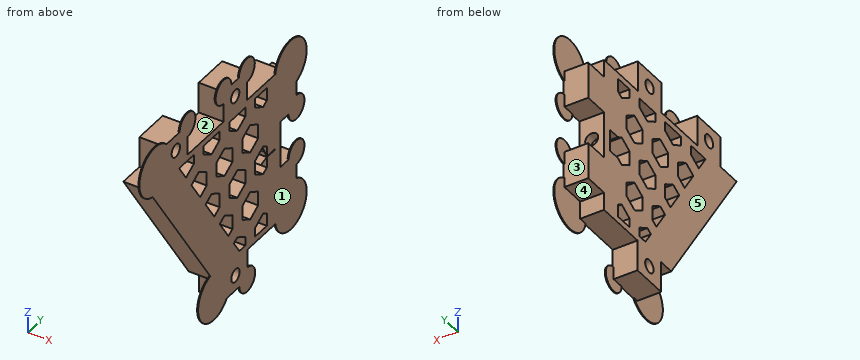
from build123d import *

# Parameters (mm, degrees)
HONEYCOMB_W      = 109
HONEYCOMB_H      = 99.592922
EXTRUDE002_DEPTH = 8
PAD002_DEPTH     = 8
PAD001_DEPTH     = 5.1
PAD_DEPTH        = 8
SKETCH001_W      = 8.1
SKETCH001_H      = 10
SKETCH001_W_2    = 18.2
SKETCH001_W_3    = 5.1
SKETCH001_W_4    = 8
SKETCH001_H_2    = 15.2
POCKET_DEPTH     = 8.001
SKETCH002_R      = 2.1
POCKET001_DEPTH  = 8.001
SKETCH004_R      = 2.1
POCKET002_DEPTH  = 7
SKETCH006_R      = 8
SKETCH006_R_2    = 4
PAD003_DEPTH     = 0.3


with BuildPart() as extrude002:
    # Honeycomb → Extrude002 (new body)
    with BuildSketch(Plane(origin=(0, 0, -0.165735), x_dir=(0, -1, 0), z_dir=(1, 0, 0))):
        with Locations((0, -0.165735)):
            Rectangle(HONEYCOMB_W, HONEYCOMB_H)
        Polygon((41.5, -37.26049), (45.5, -34.951089), (49.5, -37.26049), (49.5, -41.879292), (45.5, -44.188693), (41.5, -41.879292), align=None, mode=Mode.SUBTRACT)
        Polygon((28.5, -37.26049), (32.5, -34.951089), (36.5, -37.26049), (36.5, -41.879292), (32.5, -44.188693), (28.5, -41.879292), align=None, mode=Mode.SUBTRACT)
        Polygon((15.5, -37.26049), (19.5, -34.951089), (23.5, -37.26049), (23.5, -41.879292), (19.5, -44.188693), (15.5, -41.879292), align=None, mode=Mode.SUBTRACT)
        Polygon((2.5, -37.26049), (6.5, -34.951089), (10.5, -37.26049), (10.5, -41.879292), (6.5, -44.188693), (2.5, -41.879292), align=None, mode=Mode.SUBTRACT)
        Polygon((-10.5, -37.26049), (-6.5, -34.951089), (-2.5, -37.26049), (-2.5, -41.879292), (-6.5, -44.188693), (-10.5, -41.879292), align=None, mode=Mode.SUBTRACT)
        Polygon((-23.5, -37.26049), (-19.5, -34.951089), (-15.5, -37.26049), (-15.5, -41.879292), (-19.5, -44.188693), (-23.5, -41.879292), align=None, mode=Mode.SUBTRACT)
        Polygon((-36.5, -37.26049), (-32.5, -34.951089), (-28.5, -37.26049), (-28.5, -41.879292), (-32.5, -44.188693), (-36.5, -41.879292), align=None, mode=Mode.SUBTRACT)
        Polygon((-49.5, -37.26049), (-45.5, -34.951089), (-41.5, -37.26049), (-41.5, -41.879292), (-45.5, -44.188693), (-49.5, -41.879292), align=None, mode=Mode.SUBTRACT)
        Polygon((35, -26.00216), (39, -23.692759), (43, -26.00216), (43, -30.620962), (39, -32.930363), (35, -30.620962), align=None, mode=Mode.SUBTRACT)
        Polygon((22, -26.00216), (26, -23.692759), (30, -26.00216), (30, -30.620962), (26, -32.930363), (22, -30.620962), align=None, mode=Mode.SUBTRACT)
        Polygon((9, -26.00216), (13, -23.692759), (17, -26.00216), (17, -30.620962), (13, -32.930363), (9, -30.620962), align=None, mode=Mode.SUBTRACT)
        Polygon((-4, -26.00216), (0, -23.692759), (4, -26.00216), (4, -30.620962), (0, -32.930363), (-4, -30.620962), align=None, mode=Mode.SUBTRACT)
        Polygon((-17, -26.00216), (-13, -23.692759), (-9, -26.00216), (-9, -30.620962), (-13, -32.930363), (-17, -30.620962), align=None, mode=Mode.SUBTRACT)
        Polygon((-30, -26.00216), (-26, -23.692759), (-22, -26.00216), (-22, -30.620962), (-26, -32.930363), (-30, -30.620962), align=None, mode=Mode.SUBTRACT)
        Polygon((-43, -26.00216), (-39, -23.692759), (-35, -26.00216), (-35, -30.620962), (-39, -32.930363), (-43, -30.620962), align=None, mode=Mode.SUBTRACT)
        Polygon((41.5, -14.743829), (45.5, -12.434428), (49.5, -14.743829), (49.5, -19.362632), (45.5, -21.672033), (41.5, -19.362632), align=None, mode=Mode.SUBTRACT)
        Polygon((28.5, -14.743829), (32.5, -12.434428), (36.5, -14.743829), (36.5, -19.362632), (32.5, -21.672033), (28.5, -19.362632), align=None, mode=Mode.SUBTRACT)
        Polygon((15.5, -14.743829), (19.5, -12.434428), (23.5, -14.743829), (23.5, -19.362632), (19.5, -21.672033), (15.5, -19.362632), align=None, mode=Mode.SUBTRACT)
        Polygon((2.5, -14.743829), (6.5, -12.434428), (10.5, -14.743829), (10.5, -19.362632), (6.5, -21.672033), (2.5, -19.362632), align=None, mode=Mode.SUBTRACT)
        Polygon((-10.5, -14.743829), (-6.5, -12.434428), (-2.5, -14.743829), (-2.5, -19.362632), (-6.5, -21.672033), (-10.5, -19.362632), align=None, mode=Mode.SUBTRACT)
        Polygon((-23.5, -14.743829), (-19.5, -12.434428), (-15.5, -14.743829), (-15.5, -19.362632), (-19.5, -21.672033), (-23.5, -19.362632), align=None, mode=Mode.SUBTRACT)
        Polygon((-36.5, -14.743829), (-32.5, -12.434428), (-28.5, -14.743829), (-28.5, -19.362632), (-32.5, -21.672033), (-36.5, -19.362632), align=None, mode=Mode.SUBTRACT)
        Polygon((-49.5, -14.743829), (-45.5, -12.434428), (-41.5, -14.743829), (-41.5, -19.362632), (-45.5, -21.672033), (-49.5, -19.362632), align=None, mode=Mode.SUBTRACT)
        Polygon((35, -3.485499), (39, -1.176098), (43, -3.485499), (43, -8.104301), (39, -10.413702), (35, -8.104301), align=None, mode=Mode.SUBTRACT)
        Polygon((22, -3.485499), (26, -1.176098), (30, -3.485499), (30, -8.104301), (26, -10.413702), (22, -8.104301), align=None, mode=Mode.SUBTRACT)
        Polygon((9, -3.485499), (13, -1.176098), (17, -3.485499), (17, -8.104301), (13, -10.413702), (9, -8.104301), align=None, mode=Mode.SUBTRACT)
        Polygon((-4, -3.485499), (0, -1.176098), (4, -3.485499), (4, -8.104301), (0, -10.413702), (-4, -8.104301), align=None, mode=Mode.SUBTRACT)
        Polygon((-17, -3.485499), (-13, -1.176098), (-9, -3.485499), (-9, -8.104301), (-13, -10.413702), (-17, -8.104301), align=None, mode=Mode.SUBTRACT)
        Polygon((-30, -3.485499), (-26, -1.176098), (-22, -3.485499), (-22, -8.104301), (-26, -10.413702), (-30, -8.104301), align=None, mode=Mode.SUBTRACT)
        Polygon((-43, -3.485499), (-39, -1.176098), (-35, -3.485499), (-35, -8.104301), (-39, -10.413702), (-43, -8.104301), align=None, mode=Mode.SUBTRACT)
        Polygon((41.5, 7.772831), (45.5, 10.082232), (49.5, 7.772831), (49.5, 3.154029), (45.5, 0.844628), (41.5, 3.154029), align=None, mode=Mode.SUBTRACT)
        Polygon((28.5, 7.772831), (32.5, 10.082232), (36.5, 7.772831), (36.5, 3.154029), (32.5, 0.844628), (28.5, 3.154029), align=None, mode=Mode.SUBTRACT)
        Polygon((15.5, 7.772831), (19.5, 10.082232), (23.5, 7.772831), (23.5, 3.154029), (19.5, 0.844628), (15.5, 3.154029), align=None, mode=Mode.SUBTRACT)
        Polygon((2.5, 7.772831), (6.5, 10.082232), (10.5, 7.772831), (10.5, 3.154029), (6.5, 0.844628), (2.5, 3.154029), align=None, mode=Mode.SUBTRACT)
        Polygon((-10.5, 7.772831), (-6.5, 10.082232), (-2.5, 7.772831), (-2.5, 3.154029), (-6.5, 0.844628), (-10.5, 3.154029), align=None, mode=Mode.SUBTRACT)
        Polygon((-23.5, 7.772831), (-19.5, 10.082232), (-15.5, 7.772831), (-15.5, 3.154029), (-19.5, 0.844628), (-23.5, 3.154029), align=None, mode=Mode.SUBTRACT)
        Polygon((-36.5, 7.772831), (-32.5, 10.082232), (-28.5, 7.772831), (-28.5, 3.154029), (-32.5, 0.844628), (-36.5, 3.154029), align=None, mode=Mode.SUBTRACT)
        Polygon((-49.5, 7.772831), (-45.5, 10.082232), (-41.5, 7.772831), (-41.5, 3.154029), (-45.5, 0.844628), (-49.5, 3.154029), align=None, mode=Mode.SUBTRACT)
        Polygon((35, 19.031161), (39, 21.340562), (43, 19.031161), (43, 14.412359), (39, 12.102958), (35, 14.412359), align=None, mode=Mode.SUBTRACT)
        Polygon((22, 19.031161), (26, 21.340562), (30, 19.031161), (30, 14.412359), (26, 12.102958), (22, 14.412359), align=None, mode=Mode.SUBTRACT)
        Polygon((9, 19.031161), (13, 21.340562), (17, 19.031161), (17, 14.412359), (13, 12.102958), (9, 14.412359), align=None, mode=Mode.SUBTRACT)
        Polygon((-4, 19.031161), (0, 21.340562), (4, 19.031161), (4, 14.412359), (0, 12.102958), (-4, 14.412359), align=None, mode=Mode.SUBTRACT)
        Polygon((-17, 19.031161), (-13, 21.340562), (-9, 19.031161), (-9, 14.412359), (-13, 12.102958), (-17, 14.412359), align=None, mode=Mode.SUBTRACT)
        Polygon((-30, 19.031161), (-26, 21.340562), (-22, 19.031161), (-22, 14.412359), (-26, 12.102958), (-30, 14.412359), align=None, mode=Mode.SUBTRACT)
        Polygon((-43, 19.031161), (-39, 21.340562), (-35, 19.031161), (-35, 14.412359), (-39, 12.102958), (-43, 14.412359), align=None, mode=Mode.SUBTRACT)
        Polygon((41.5, 30.289492), (45.5, 32.598893), (49.5, 30.289492), (49.5, 25.670689), (45.5, 23.361288), (41.5, 25.670689), align=None, mode=Mode.SUBTRACT)
        Polygon((28.5, 30.289492), (32.5, 32.598893), (36.5, 30.289492), (36.5, 25.670689), (32.5, 23.361288), (28.5, 25.670689), align=None, mode=Mode.SUBTRACT)
        Polygon((15.5, 30.289492), (19.5, 32.598893), (23.5, 30.289492), (23.5, 25.670689), (19.5, 23.361288), (15.5, 25.670689), align=None, mode=Mode.SUBTRACT)
        Polygon((2.5, 30.289492), (6.5, 32.598893), (10.5, 30.289492), (10.5, 25.670689), (6.5, 23.361288), (2.5, 25.670689), align=None, mode=Mode.SUBTRACT)
        Polygon((-10.5, 30.289492), (-6.5, 32.598893), (-2.5, 30.289492), (-2.5, 25.670689), (-6.5, 23.361288), (-10.5, 25.670689), align=None, mode=Mode.SUBTRACT)
        Polygon((-23.5, 30.289492), (-19.5, 32.598893), (-15.5, 30.289492), (-15.5, 25.670689), (-19.5, 23.361288), (-23.5, 25.670689), align=None, mode=Mode.SUBTRACT)
        Polygon((-36.5, 30.289492), (-32.5, 32.598893), (-28.5, 30.289492), (-28.5, 25.670689), (-32.5, 23.361288), (-36.5, 25.670689), align=None, mode=Mode.SUBTRACT)
        Polygon((-49.5, 30.289492), (-45.5, 32.598893), (-41.5, 30.289492), (-41.5, 25.670689), (-45.5, 23.361288), (-49.5, 25.670689), align=None, mode=Mode.SUBTRACT)
        Polygon((35, 41.547822), (39, 43.857223), (43, 41.547822), (43, 36.92902), (39, 34.619619), (35, 36.92902), align=None, mode=Mode.SUBTRACT)
        Polygon((22, 41.547822), (26, 43.857223), (30, 41.547822), (30, 36.92902), (26, 34.619619), (22, 36.92902), align=None, mode=Mode.SUBTRACT)
        Polygon((9, 41.547822), (13, 43.857223), (17, 41.547822), (17, 36.92902), (13, 34.619619), (9, 36.92902), align=None, mode=Mode.SUBTRACT)
        Polygon((-4, 41.547822), (0, 43.857223), (4, 41.547822), (4, 36.92902), (0, 34.619619), (-4, 36.92902), align=None, mode=Mode.SUBTRACT)
        Polygon((-17, 41.547822), (-13, 43.857223), (-9, 41.547822), (-9, 36.92902), (-13, 34.619619), (-17, 36.92902), align=None, mode=Mode.SUBTRACT)
        Polygon((-30, 41.547822), (-26, 43.857223), (-22, 41.547822), (-22, 36.92902), (-26, 34.619619), (-30, 36.92902), align=None, mode=Mode.SUBTRACT)
        Polygon((-43, 41.547822), (-39, 43.857223), (-35, 41.547822), (-35, 36.92902), (-39, 34.619619), (-43, 36.92902), align=None, mode=Mode.SUBTRACT)
    extrude(amount=EXTRUDE002_DEPTH)


with BuildPart() as extrude002_1:
    # Extrude002 placement: moved
    add(extrude002.part.moved(Location((0, 1.1, 5.6))))


with BuildPart() as common:
    # Sketch005 → Pad002 (new body)
    with BuildSketch(Plane.YZ):
        Polygon((22.5, 23.15), (22.5, -23.15), (8.5944, -23.15), (-21.8273, 23.15), align=None)
    extrude(amount=PAD002_DEPTH)

    # Common: intersect Extrude002
    add(extrude002_1.part, mode=Mode.INTERSECT)


with BuildPart() as pad001:
    # Sketch003 → Pad001 (new body)
    with BuildSketch(Plane.XZ.offset(-26.5)):
        Polygon((1.96484, -3.525), (6.03516, -3.525), (8.070319, 0), (6.03516, 3.525), (0, 3.525), (0, -3.525), align=None)
    extrude(amount=PAD001_DEPTH)


with BuildPart() as obj1:
    # Sketch → Pad (new body)
    with BuildSketch(Plane.YZ):
        Polygon((-37.5, 35.15), (37.5, 35.15), (37.5, -35.15), (-4.45, -35.15), (-4.45, -25.15), (-37.5, 25.15), align=None)
        Polygon((-21.827321, 23.15), (22.5, 23.15), (22.5, -23.15), (8.594449, -23.15), align=None, mode=Mode.SUBTRACT)
    extrude(amount=PAD_DEPTH)

    # Sketch001 → Pocket (cut, through all)
    with BuildSketch(Plane.YZ.offset(8)):
        with Locations((-33.45, 30.15)):
            Rectangle(SKETCH001_W, SKETCH001_H)
        with Locations((-8.5, 30.15)):
            Rectangle(SKETCH001_W_2, SKETCH001_H)
        Polygon((37.5, 35.15), (12.4, 35.15), (12.4, 25.15), (29.5, 25.15), (29.5, 19.45), (37.5, 19.45), align=None)
        with Locations((-1.9, -30.15)):
            Rectangle(SKETCH001_W_3, SKETCH001_H)
        Polygon((12.6, -35.15), (37.5, -35.15), (37.5, -25.15), (37.5, -19.4), (29.5, -19.4), (29.5, -25.15), (12.6, -25.15), align=None)
        with Locations((33.5, 0)):
            Rectangle(SKETCH001_W_4, SKETCH001_H_2)
    extrude(amount=-POCKET_DEPTH, mode=Mode.SUBTRACT)

    # Sketch002 → Pocket001 (cut, through all)
    with BuildSketch(Plane.YZ.offset(8)):
        with Locations((-23.5, 30.15)):
            Circle(SKETCH002_R)
        with Locations((6.5, 30.15)):
            Circle(SKETCH002_R)
        with Locations((6.625, -30.15)):
            Circle(SKETCH002_R)
    extrude(amount=-POCKET001_DEPTH, mode=Mode.SUBTRACT)

    # Cut: cut Pad001
    add(pad001.part, mode=Mode.SUBTRACT)

    # Sketch004 → Pocket002 (cut)
    with BuildSketch(Plane(origin=(0, 29.5, 0), x_dir=(-1, 0, 0), z_dir=(0, 1, 0))):
        with Locations((-4, 0)):
            Circle(SKETCH004_R)
    extrude(amount=-POCKET002_DEPTH, mode=Mode.SUBTRACT)

    # Fusion: union Common
    add(common.part)

    # Sketch006 → Pad003 (new body)
    with BuildSketch(Plane.YZ.offset(8)):
        with Locations((34.628638, 23.70913)):
            Circle(SKETCH006_R)
        with Locations((34.628638, -23.70913)):
            Circle(SKETCH006_R)
        with Locations((-33.930172, 29.614136)):
            Circle(SKETCH006_R)
        with Locations((-4.250326, -30.439821)):
            Circle(SKETCH006_R)
        with Locations((-17.6, 35.15)):
            Circle(SKETCH006_R_2)
        with Locations((0.6, 35.15)):
            Circle(SKETCH006_R_2)
        with Locations((12.4, 35.15)):
            Circle(SKETCH006_R_2)
        with Locations((12.6, -35.15)):
            Circle(SKETCH006_R_2)
        with Locations((37.5, 7.6)):
            Circle(SKETCH006_R_2)
        with Locations((37.5, -7.6)):
            Circle(SKETCH006_R_2)
    extrude(amount=-PAD003_DEPTH)


solid = obj1.part
Model file for the job. Use its own axes, mm. Face numbers are marked on the shaded views. A direction names the side the tool comes from. Give positions to 0.01 mm unless a question says otherwise; leave off trailing zeros. Order: outer loops, then holes, each group sorted by start corner. A loop starts at its lowest first (then second) coordinate and runs counter-clockwise, first axis right, second up. Notation, with made-up numbers: (-8, 27) - (20, 27) arc R18 cw to (20, 43) - close; hole circle Ø6 at (37.5, 27). An arc over 180 degrees is marked (long way). Write item = value, one per line. Start each with the question number.
1. Cut at B-B, the plane z = 30.15. List the corners of the cut face in (x, y), and give its area (3 significant figures).
2. Which spindle directions (+Z, -Z, +X, -X, +Y, -Y) get a long thin tool onto all of the face, cutting with end or side? Do the marked faces 4 and 5. Say none if no direction does.
3. Two-plate mould, pull along Y, no slides. Class the marked faces 1, 2 and 3: pulls with the +Y half, pulls with the -Y half, needs draft (parallel to the pull), parting line crosses it, or undercut.
4. Probe line 1 along Y through (x, z) = (6, -14); line 2 along Y through (x, z) = (1.75, -22); line 3 along Z through (x, y) = (1.5, 25.5) (3 decimals). List the from-to ranges inside material, lowest first.
5. Cut at C-C, the plane x = 3.25. State how many separate pieces and enclosed holes the cut face has, and give its area (3 significant figures).
6. Drop flat-ended pins along their axis: P1, Ø4, axis at x = 7, z = -0.5, coming from the +Y side; P2, Ø4, axis at x = 5.5, y = -3.5, coming from the -Z side; P3, Ø5, axis at y = 31, z = -29, coming from the -X side; P4, Ø7, axis at y = -35, z = 28.5, coming from the -X side. Give the stop position or say it passes through.
7. Cut at A-A, the plane z = -30.15. List the corners of the cut face in (x, y) (3 decimals).
Taken from the geometry:
q1.outline = (0, -29.4) - (7.7, -29.4) - (7.7, -41.91) - (8, -41.91) - (8, -25.6) - (0, -25.6) - close; (0, -21.4) - (8, -21.4) - (8, -17.6) - (0, -17.6) - close; (0, 0.6) - (8, 0.6) - (8, 4.4) - (0, 4.4) - close; (0, 8.6) - (8, 8.6) - (8, 12.4) - (0, 12.4) - close; (7.7, 29.88) - (8, 29.88) - (8, 39.37) - (7.7, 39.37) - close
q1.area = 128 mm²
q2.face_4 = -Z, -X, +Y
q2.face_5 = +Z, -Z, -X, +Y, -Y
q3.face_1 = needs draft
q3.face_2 = undercut
q3.face_3 = pulls with the +Y half
q4.line_1 = -11.78 to 2.58, 4.4 to 10.8, 17.4 to 37.5
q4.line_2 = -6.52 to 7.84, 11.6 to 16.6, 22.5 to 29.5
q4.line_3 = -25.15 to -3.525, 3.525 to 25.15
q5.separate_pieces = 1
q5.enclosed_holes = 15
q5.area = 2,470 mm²
q6.P1 = 29.5
q6.P2 = -25.15
q6.P3 = 7.7
q6.P4 = 0
q7.outline = (0, 0.65) - (7.7, 0.65) - (7.7, -12.245) - (8, -12.245) - (8, 4.525) - (0, 4.525) - close; (0, 8.725) - (8, 8.725) - (8, 12.6) - (0, 12.6) - close; (7.7, 29.884) - (8, 29.884) - (8, 39.374) - (7.7, 39.374) - close
